Verification items for the finished model (mm, model axes). A direction names the side the tool comes from. Coordinates: 2 decimals unless noted, no trailing zeros. Write each loop counter-clockwise with the first axis right and the second up, starting at its lowest first coordinate (ties: lowest second). Pieces come first, ordered by that corner, then holes. Notation, with made-up numbers: M 80,3 L 85,3 A23 ccw 85,25 Z; hole C 2.25,58 d5. An arc over 180 degrees is marked long. Answer in a Markdown table with one row per item.
from build123d import *
from build123d.topology import SkipClean

# Parameters (mm, degrees)
BOSS_EXTRUDE1_DEPTH = 44.45
BOSS_EXTRUDE2_DEPTH = 25.4


with BuildPart() as part:
    # Sketch1 → Boss-Extrude1 (new body)
    with BuildSketch(Plane(origin=(0, 0, 0), x_dir=(1, 0, 0), z_dir=(0, 1, 0))):
        with BuildLine():
            Line((-4.099560952, 3), (4.099560952, 3))
            ThreePointArc((4.099560952, 3), (0, -5.08), (-4.099560952, 3))
        make_face()
    extrude(amount=BOSS_EXTRUDE1_DEPTH)

    # Sketch3 → Boss-Extrude2 (add)
    with SkipClean():  # the faces are left unmerged after this step: merging them gives an invalid solid
        with BuildSketch(Plane.XZ):
            with BuildLine():
                Line((-4.099560952, -3), (4.099560952, -3))
                ThreePointArc((4.099560952, -3), (0, -5.08), (-4.099560952, -3))
            make_face()
        extrude(amount=-BOSS_EXTRUDE2_DEPTH)


solid = part.part
1) Sectioned sample at B-B (x = 2.5). Record the cut outline in (y, z), then the cut area to 3 significant figures.
Response values:
| item | result |
|---|---|
| outline | M 0,-4.42 L 25.4,-4.42 L 25.4,-3 L 44.45,-3 L 44.45,4.42 L 0,4.42 Z |
| area | 366 mm² |
2) Sectioned sample at D-D (x = 0). Record the cut outline in (y, z), then the cut area to 3 significant figures.
Response values:
| item | result |
|---|---|
| outline | M 0,-5.08 L 25.4,-5.08 L 25.4,-3 L 44.45,-3 L 44.45,5.08 L 0,5.08 Z |
| area | 412 mm² |
3) Thickness scan on L1, parallel to Z at x = -3, y = 32.5; L2, parallel to X at y = 26.5, z = -0.25; L3, parallel to Y at x = -0.5, z = -4. Record the ranges inside material, lowest first. Write a range as [from, to].
Response values:
| item | result |
|---|---|
| L1 | z = [-3, 4.1] |
| L2 | x = [-5.07, 5.07] |
| L3 | y = [0, 25.4] |
4) Depth check by flat-ended pin: pin 1 (5 mm diameter, centred on x = 1.5, y = 27.5, fed in from +Z); pin 2 (1.5 mm diameter, centred on y = 15, z = 2.5, fed in from +X); pin 3 (0.6 mm diameter, centred on x = 1.5, z = -4.5, fed in from +Y); pin 4 (5 mm diameter, centred on x = 0.5, y = 32.5, fed in from -Z). Enter the tip coordinate at first touch or a pass-through.
Response values:
| item | result |
|---|---|
| pin 1 | stops at z = 5.08 |
| pin 2 | stops at x = 4.77 |
| pin 3 | stops at y = 25.4 |
| pin 4 | stops at z = -3 |
5) Sectioned sample at C-C (y = 39). Record the cut outline in (x, z), then the cut area to 3 significant figures.
Response values:
| item | result |
|---|---|
| outline | M -4.1,-3 L 4.1,-3 A5.08 ccw long Z |
| area | 69.1 mm² |
6) Tool access check on faces 1 (the face through (0, 35, -3)), 2 (the face through (0, 0, 0)). Record the directions out of +Z, -Z, +X, -X, +Y, -Y that give a thin tool (end or side, any length) a straight path to the whole face; none if there is none.
Response values:
| item | result |
|---|---|
| face 1 | -Z, +X, -X, +Y |
| face 2 | +Z, -Z, +X, -X, -Y |
7) Sectioned sample at A-A (z = 3). Record the cut outline in (x, y).
Response values:
| item | result |
|---|---|
| outline | M -4.1,0 L 4.1,0 L 4.1,44.45 L -4.1,44.45 Z |
